Autodesk Inventor part; units mm, degrees
ref_plane "YZ Plane" through (0, 0, 0) normal (1, 0, 0) x (0, 1, 0)
ref_plane "XZ Plane" through (0, 0, 0) normal (0, 1, 0) x (-1, 0, 0)
ref_plane "XY Plane" through (0, 0, 0) normal (0, 0, 1) x (1, 0, 0)
sketch "Sketch1" plane through (0, 0, 0) normal (0, 1, 0) x (-1, 0, 0)
  line L0 (0, 0) -> (0, -23)
  line L1 (0, -23) -> (20, -23)
  line L2 (20, -23) -> (20, 0)
  line L3 (16.0214, -11.5) -> (3.8301, -11.5) construction
  circle A0 centre (12.5, -11.5) radius 0.5
  line L4 (20, 0) -> (0, 0)
  dimension "d0" = 23
  dimension "d2" = 1
  dimension "d3" = 7.5
  dimension "d10" = 20
extrude "Extrusion3" add sketch "Sketch1" along normal blind 1.5
properties part number "Distance_test_adaptor_circle_1mm"
Geometry: final body of the model. Coordinates: model frame, mm. Coordinates: 2 decimals unless noted, no trailing zeros. Order: outer loops, then holes, each group sorted by start corner. A loop starts at its lowest first (then second) coordinate and runs counter-clockwise, first axis right, second up. Notation, with made-up numbers: (-30.5, -18.5) - (4.5, -18.5) arc R25 cw to (4.5, -0.5) - close; hole circle Ø8 at (18.25, -7.5). An arc over 180 degrees is marked (long way). Return JSON: item names as keys, results as strings. Group by question number.
1. Cut plane A-A (x = -12.5). Output: boundary loops of the cut face in (y, z).
2. Material intervals for line 1 along Z through (x, y) = (-12.5, 1), sorted ascending. Write a range as [from, to].
3. Cut plane B-B (z = -11.5). Output: boundary loops of the cut face in (x, y).
4. Pull-direction query (X, two-part tool) for faces 1 (the face through (-12.731, 0.74, -11.056)), 2 (the face through (-20, 1, -12)), 3 (the face through (-10, 1, 0)); classes: pulls with the +X half, pulls with the -X half, needs draft (parallel to the pull), parting line crosses it, or undercut.
Resolved:
{
 "1": {"outline": "(0, -23) - (1.5, -23) - (1.5, -12) - (0, -12) - close; (0, -11) - (1.5, -11) - (1.5, 0) - (0, 0) - close"},
 "2": {"line 1": "z = [-23, -12], [-11, 0]"},
 "3": {"outline": "(-20, 0) - (-13, 0) - (-13, 1.5) - (-20, 1.5) - close; (-12, 0) - (0, 0) - (0, 1.5) - (-12, 1.5) - close"},
 "4": {"face 1": "undercut", "face 2": "pulls with the -X half", "face 3": "needs draft"}
}
